Can you work these out from the model? Positions are in its coordinate system, mm. Coordinates: 2 decimals unless noted, no trailing zeros. Order: outer loops, then holes, each group sorted by start corner. A loop starts at its lowest first (then second) coordinate and runs counter-clockwise, first axis right, second up. Notation, with made-up numbers: (73.5, 4) - (96.5, 4) arc R23 cw to (96.5, 42) - close; hole circle Ø2 at (49.5, -39). An arc over 180 degrees is marked (long way). Use a Markdown table: item, result. Add a question column.
(1) I want a section at C-C (z = 46.5). List the corners of the cut face in (x, y) for me, and give its area (3 significant figures).
(2) If I drill on L1, parallel to Z at x = 80, y = -2.8; L2, parallel to X at y = -3.55, z = 45; L3, parallel to X at y = -0.95, z = -71, over which ranges is the centre line in solid material (lowest first)? Write a range as [from, to].
(3) I want a section at A-A (y = -2.95). List the corners of the cut face in (x, z) for me, and give its area (3 significant figures).
(4) For pin 1 Ø2 at (x, y) = (83.5, -2) entering from +Z, with a flat end and sliding along its axis, tell me the tip position at first contact or that it passes through.
(5) We'd pull the mould along Z, two halves only. Please class faces 1 (the flat face through (120, -2, -11)), 2 (the flat face through (-1, -2, -91)), 3 (the cylindrical face through (85.11, -2.46, 59.01)): pulls with the +Z half, pulls with the -Z half, needs draft (parallel to the pull), parting line crosses it, or undercut.
(6) I want a section at B-B (x = -95). List the corners of the cut face in (y, z) for me.
```python
from build123d import *

# Parameters (mm, degrees)
F0_R     = 9.5
F1_DEPTH = 5
F2_R     = 20


with BuildPart() as f1:
    # F0 (on Front) → F1 (new body)
    with BuildSketch(Plane.XZ):
        with BuildLine():
            ThreePointArc((-85.5, -66), (-95, -56.5), (-104.5, -66))
            ThreePointArc((-104.5, -66), (-95, -75.5), (-85.5, -66))
        make_face()
        with Locations((95, -66)):
            Circle(F0_R)
        Polygon((120, 51), (80, 91), (-80, 91), (-120, 51), (-120, -66), (-120, -91), (120, -91), (120, -66), align=None)
        with BuildLine():
            ThreePointArc((-85.5, -66), (-95, -75.5), (-104.5, -66))
            ThreePointArc((-104.5, -66), (-95, -56.5), (-85.5, -66))
        make_face(mode=Mode.SUBTRACT)
        with Locations((95, -66)):
            Circle(F0_R, mode=Mode.SUBTRACT)
        with Locations((-80, 51)):
            Circle(F0_R, mode=Mode.SUBTRACT)
        with Locations((80, 51)):
            Circle(F0_R, mode=Mode.SUBTRACT)
    extrude(amount=F1_DEPTH)

    # F2
    f2_edges = [f1.edges().sort_by_distance(p)[0] for p in [
        (-120, -2.5, -91),
        (120, -2.5, -91),
    ]]
    fillet(f2_edges, radius=F2_R)


solid = f1.part
```
Answers follow:
| question | item | result |
|---|---|---|
| 1 | outline | (-120, -5) - (-88.37, -5) - (-88.37, 0) - (-120, 0) - close; (-71.63, -5) - (71.63, -5) - (71.63, 0) - (-71.63, 0) - close; (88.37, -5) - (120, -5) - (120, 0) - (88.37, 0) - close |
| 1 | area | 1,030 mm² |
| 2 | L1 | z = [-91, 41.5], [60.5, 91] |
| 2 | L2 | x = [-120, -87.37], [-72.63, 72.63], [87.37, 120] |
| 2 | L3 | x = [-120, -103.08], [-86.92, 86.92], [103.08, 120] |
| 3 | outline | (-120, -71) arc R20 ccw to (-100, -91) - (100, -91) arc R20 ccw to (120, -71) - (120, 51) - (80, 91) - (-80, 91) - (-120, 51) - close; hole circle Ø19 at (-95, -66); hole circle Ø19 at (-80, 51); hole circle Ø19 at (80, 51); hole circle Ø19 at (95, -66) |
| 3 | area | 40,800 mm² |
| 4 | pin 1 | stops at z = 88.5 |
| 5 | face 1 | needs draft |
| 5 | face 2 | pulls with the -Z half |
| 5 | face 3 | undercut |
| 6 | outline | (-5, -91) - (0, -91) - (0, -75.5) - (-5, -75.5) - close; (-5, -56.5) - (0, -56.5) - (0, 76) - (-5, 76) - close |
